The model under review builds one solid part; all positions refer to its coordinate system, in mm. Face numbers are marked on the shaded views. A direction names the side the tool comes from. Coordinates: 2 decimals unless noted, no trailing zeros. Order: outer loops, then holes, each group sorted by start corner. A loop starts at its lowest first (then second) coordinate and runs counter-clockwise, first axis right, second up. Notation, with made-up numbers: (81.25, -13) - (129.25, -13) arc R21 ccw to (129.25, 3) - close; hole circle Ø8 at (7.25, 25.5). An arc over 180 degrees is marked (long way). Answer in a Markdown table with one row per item.
```python
from build123d import *

# Parameters (mm, degrees)
BOSS_EXTRU_1_DEPTH      = 5
ESQUISSE2_R             = 1.6
ENL_V_MAT_EXTRU_1_DEPTH = 71.691230008
CONG_1_R                = 1
CONG_2_R                = 1


with BuildPart() as part:
    # Esquisse1 → Boss.-Extru.1 (new body)
    with BuildSketch(Plane.XY):
        with BuildLine():
            Line((0, 0), (70, 0))
            Line((70, 0), (70, 2))
            Line((70, 2), (56.447221814, 2))
            Line((56.447221814, 2), (56.447221814, 10.5))
            Line((56.447221814, 10.5), (54.447221814, 10.5))
            ThreePointArc((54.447221814, 10.5), (45, 2), (35.552778186, 10.5))
            Line((35.552778186, 10.5), (34.447221814, 10.5))
            ThreePointArc((34.447221814, 10.5), (25, 2), (15.552778186, 10.5))
            Line((15.552778186, 10.5), (13.552778186, 10.5))
            Line((13.552778186, 10.5), (13.552778186, 2))
            Line((13.552778186, 2), (0, 2))
            Line((0, 2), (0, 0))
        make_face()
    extrude(amount=BOSS_EXTRU_1_DEPTH)

    # Esquisse2 → Enlèv. mat.-Extru.1 (cut, through all)
    with BuildSketch(Plane(origin=(0, 2, 0), x_dir=(1, 0, 0), z_dir=(0, 1, 0))):
        with Locations(Location((6.776389093, -2.5, 0), (0, 0, 270))):
            Circle(ESQUISSE2_R)
        with Locations(Location((61.776389093, -2.5, 0), (0, 0, 90))):
            Circle(ESQUISSE2_R)
    extrude(amount=-ENL_V_MAT_EXTRU_1_DEPTH, mode=Mode.SUBTRACT)

    # Congé1
    cong_1_edges = [part.edges().sort_by_distance(p)[0] for p in [
        (13.552778186, 2, 2.5),
    ]]
    fillet(cong_1_edges, radius=CONG_1_R)

    # Congé2
    # the kernel refuses this fillet: 1 mm, written as the material it adds along each edge
    with BuildSketch(Plane(origin=(56.447221814, 2, 0), x_dir=(1, 0, 0), z_dir=(0, 0, 1))) as cong_2_piece_1:
        with BuildLine():
            CenterArc((CONG_2_R, CONG_2_R), CONG_2_R, 180, 90)
            Line((0, CONG_2_R), (0, 0))
            Line((0, 0), (CONG_2_R, 0))
        make_face()
    extrude(amount=5)
    # the kernel refuses this fillet: 1 mm, written as the material it takes off along each edge
    with BuildSketch(Plane(origin=(13.552778186, 10.5, -2.5), x_dir=(0, -1, 0), z_dir=(0, 0, 1)), Plane(origin=(56.447221814, 10.5, -2.5), x_dir=(-1, 0, 0), z_dir=(0, 0, 1))) as cong_2_2_piece_1:
        with BuildLine():
            CenterArc((CONG_2_R, CONG_2_R), CONG_2_R, 180, 90)
            Line((0, CONG_2_R), (0, 0))
            Line((0, 0), (CONG_2_R, 0))
        make_face()
    extrude(amount=10, mode=Mode.SUBTRACT)
    with BuildSketch(Plane(origin=(15.552778186, 10.5, -2.151355625), x_dir=(-1, 0, 0), z_dir=(0, 0, 1)), Plane(origin=(35.552778186, 10.5, -2.151355625), x_dir=(-1, 0, 0), z_dir=(0, 0, 1))) as cong_2_2_piece_2:
        with BuildLine():
            CenterArc((0.86054225, 1), CONG_2_R, 190.980575428, 79.019424572)
            ThreePointArc((-0.121149565, 0.80952381), (-0.05185196, 0.406067322), (0, 0))
            Line((0, 0), (0.86054225, 0))
        make_face()
    extrude(amount=9.302711251, mode=Mode.SUBTRACT)
    with BuildSketch(Plane(origin=(34.447221814, 10.5, -2.151355625), x_dir=(-0.1480070865029111, -0.9889863003828312, 0), z_dir=(0, 0, 1)), Plane(origin=(54.447221814, 10.5, -2.151355625), x_dir=(-0.1480070865029111, -0.9889863003828312, 0), z_dir=(0, 0, 1))) as cong_2_2_piece_3:
        with BuildLine():
            CenterArc((0.861619949, 0.999071583), CONG_2_R, 188.511451923, 79.019424572)
            Line((-0.127366351, 0.851064496), (0, 0))
            ThreePointArc((0, 0), (0.409269476, 0.008819963), (0.818538952, 0))
        make_face()
    extrude(amount=9.302711251, mode=Mode.SUBTRACT)


solid = part.part
```
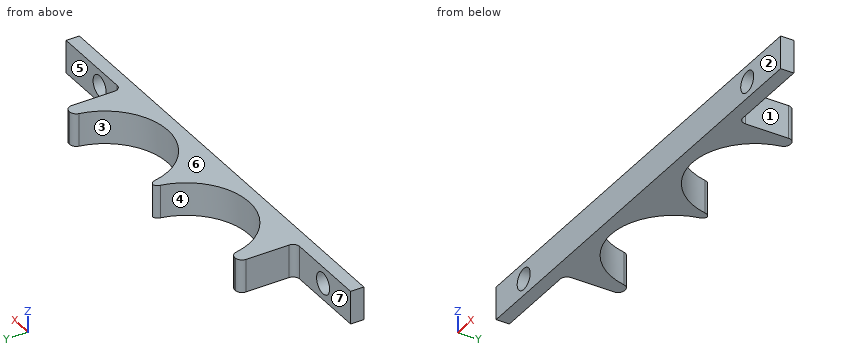
Item 1: Tool access review of the marked faces 5, 6 and 7: name each direction out of +Z, -Z, +X, -X, +Y, -Y from which nothing blocks a thin tool from reaching the whole face with its end or side.
Check values:
| item | result |
|---|---|
| face 5 | +Z, -Z, +X, +Y |
| face 6 | +Z, +X, -X, +Y, -Y |
| face 7 | +Z, -Z, -X, +Y |
Item 2: We need section C-C, the plane x = 51. Write out the cut boundary in (y, z).
Check values:
| item | result |
|---|---|
| outline | (0, 0) - (4.13, 0) - (4.13, 5) - (0, 5) - close |
Item 3: We need section A-A, the plane z = 1.85. Write out the cut boundary in (x, y), then the cut area to 3 significant figures.
Check values:
| item | result |
|---|---|
| outline | (0, 0) - (5.31, 0) - (5.31, 2) - (0, 2) - close; (8.24, 0) - (60.31, 0) - (60.31, 2) - (57.45, 2) arc R1 cw to (56.45, 3) - (56.45, 9.5) arc R1 ccw to (55.45, 10.5) - (55.31, 10.5) arc R1 ccw to (54.33, 9.69) arc R9.5 cw to (35.67, 9.69) arc R1 ccw to (35, 10.45) arc R1 ccw to (34.33, 9.69) arc R9.5 cw to (15.67, 9.69) arc R1 ccw to (14.69, 10.5) - (14.55, 10.5) arc R1 ccw to (13.55, 9.5) - (13.55, 3) arc R1 cw to (12.55, 2) - (8.24, 2) - close; (63.24, 0) - (70, 0) - (70, 2) - (63.24, 2) - close |
| area | 247 mm^2 |
Item 4: We need section B-B, the plane y = 7.5. Write out the cut boundary in (x, z), then the cut area to 3 significant figures.
Check values:
| item | result |
|---|---|
| outline | (13.55, 0) - (16.38, 0) - (16.38, 5) - (13.55, 5) - close; (33.62, 0) - (36.38, 0) - (36.38, 5) - (33.62, 5) - close; (53.62, 0) - (56.45, 0) - (56.45, 5) - (53.62, 5) - close |
| area | 42.1 mm^2 |
Item 5: To check wall thickness, follow line 1 (X direction, y = 1.3, z = 2.5); line 2 (X direction, y = 7.25, z = 2.9); line 3 (Y direction, x = 12, z = 1.9). State the ranges of each line that lie inside material, in increasing order. Write a range as from..to.
Check values:
| item | result |
|---|---|
| line 1 | 0..5.18, 8.38..60.18, 63.38..70 |
| line 2 | 13.55..16.5, 33.5..36.5, 53.5..56.45 |
| line 3 | 0..2 |
Item 6: Clearance check with flat-ended pins moving along their axes: pin 1 Ø2 at (x, z) = (59.5, 3.5) entering from -Y; pin 2 Ø1 at (y, z) = (3.5, 4) entering from +X. State where each tip first meets the part, or that it passes through.
Check values:
| item | result |
|---|---|
| pin 1 | y = 0 |
| pin 2 | x = 56.45 |
Item 7: Mouldability with a two-part tool opening along X and no side actions: class the marked faces 1, 2, 3 and 4 as +X half, -X half, draft (parallel to the pull), parting line (faces both ways), or undercut.
Check values:
| item | result |
|---|---|
| face 1 | +X half |
| face 2 | draft |
| face 3 | undercut |
| face 4 | undercut |
